Design review of the part built by this model. Coordinates are the model's own, in mm. A direction names the side the tool comes from. Give positions to 0.01 mm unless a question says otherwise; leave off trailing zeros. Loops run counter-clockwise (first coordinate to the right, second up) from the corner with the lowest first, then second, coordinate; pieces in that order, holes last. Notation, with made-up numbers: (44, -17) - (63, -17) arc R24 cw to (63, 4) - close; hole circle Ø6 at (35.25, 85.25). An arc over 180 degrees is marked (long way). Write each question's results on one line, items separated by ' | '.
from build123d import *

# Parameters (mm, degrees)
SKETCH_1_R          = 1.1303
EXTRUDE_1_DEPTH     = 1.588
FILLET_1_R          = 2
FILLET_2_R          = 2
FILLET_3_R          = 2
FILLET_4_R          = 2
SKETCH_2_W          = 12
SKETCH_2_H          = 89.95
EXTRUDE_2_DEPTH     = 1.588
CUT_EXTRUDE_1_DEPTH = 10


with BuildPart() as part:
    # 草图1 → 凸台-拉伸1 (new body)
    with BuildSketch(Plane(origin=(-0.79375, 0, 0), x_dir=(0, -1, 0), z_dir=(-1, 0, 0))):
        with BuildLine():
            Line((38.795, 5), (12.795, 5))
            ThreePointArc((12.795, 5), (11.380786438, 4.414213562), (10.795, 3))
            Line((10.795, 3), (10.795, -13))
            ThreePointArc((10.795, -13), (11.380786438, -14.414213562), (12.795, -15))
            Line((12.795, -15), (47.795, -15))
            Line((47.795, -15), (50.77, -0.039144756))
            Line((50.77, -0.039144756), (55.77, -0.039144756))
            Line((55.77, -0.039144756), (60.77, -0.039144756))
            Line((60.77, -0.039144756), (63.745, -15))
            Line((63.745, -15), (98.745, -15))
            ThreePointArc((98.745, -15), (100.159213562, -14.414213562), (100.745, -13))
            Line((100.745, -13), (100.745, 3))
            ThreePointArc((100.745, 3), (100.159213562, 4.414213562), (98.745, 5))
            Line((98.745, 5), (72.745, 5))
            Line((72.745, 5), (38.795, 5))
        make_face()
        with Locations((18.295, 0)):
            Circle(SKETCH_1_R, mode=Mode.SUBTRACT)
        with Locations((13.295, 0)):
            Circle(SKETCH_1_R, mode=Mode.SUBTRACT)
        with Locations((98.245, 0)):
            Circle(SKETCH_1_R, mode=Mode.SUBTRACT)
        with Locations((93.245, 0)):
            Circle(SKETCH_1_R, mode=Mode.SUBTRACT)
    extrude(amount=-EXTRUDE_1_DEPTH)

    # 圆角1
    fillet_1_edges = [part.edges().sort_by_distance(p)[0] for p in [
        (0.00025, -50.77, -0.039144756),
    ]]
    fillet(fillet_1_edges, radius=FILLET_1_R)

    # 圆角2
    fillet_2_edges = [part.edges().sort_by_distance(p)[0] for p in [
        (0.00025, -47.795, -15),
    ]]
    fillet(fillet_2_edges, radius=FILLET_2_R)

    # 圆角3
    fillet_3_edges = [part.edges().sort_by_distance(p)[0] for p in [
        (0.00025, -60.77, -0.039144756),
    ]]
    fillet(fillet_3_edges, radius=FILLET_3_R)

    # 圆角4
    fillet_4_edges = [part.edges().sort_by_distance(p)[0] for p in [
        (0.00025, -63.745, -15),
    ]]
    fillet(fillet_4_edges, radius=FILLET_4_R)

    # 草图2 → 凸台-拉伸2 (add)
    with BuildSketch(Plane.ZY.offset(0.79375)):
        with Locations((9, -55.77)):
            Rectangle(SKETCH_2_W, SKETCH_2_H)
        Polygon((-25, -10.795), (-25, -45.806477318), (-13.39006724, -48.115138781), (-13, -10.795), align=None)
        Polygon((-13.39006724, -63.424861219), (-25, -65.733522682), (-25, -100.745), (-13, -100.745), align=None)
    extrude(amount=-EXTRUDE_2_DEPTH)

    # 草图5 → 切除-拉伸1 (cut)
    with BuildSketch(Plane(origin=(0.79425, 0, 0), x_dir=(0, 0, -1), z_dir=(1, 0, 0))):
        Polygon((1.649077515, -50.449861219), (25, -45.806477318), (25, -39.241825321), align=None)
        Polygon((25, -72.298174679), (25, -65.733522682), (1.649077515, -61.090138781), align=None)
    extrude(amount=-CUT_EXTRUDE_1_DEPTH, mode=Mode.SUBTRACT)


solid = part.part
(1) Wall thickness on line 1 along Y through (x, z) = (-0.6, -5.5) (3 decimals); line 2 along Y through (x, z) = (0.1, -20) (3 decimals); line 3 along Z through (x, y) = (-0.05, -71): over which ranges is each line inside the solid? List them lowest first. Write a range as from..to.
Answers below:
line 1: -100.745..-62.939, -48.601..-10.795 | line 2: -100.745..-69.898, -41.642..-10.795 | line 3: -22.3..15
(2) Take a section at B-B on z = -13.5. Give the boundary of the cut face in (x, y) (3 decimals).
Answers below:
outline: (-0.794, -100.745) - (0.794, -100.745) - (0.794, -66.778) - (-0.794, -66.778) - close; (-0.794, -44.762) - (0.794, -44.762) - (0.794, -10.795) - (-0.794, -10.795) - close
(3) Tool access review of faces 4 (the flat face through (0.011, -66.616, -13.161)), 5 (the flat face through (0, -86, -25)): name each direction out of +Z, -Z, +X, -X, +Y, -Y from which nothing blocks a thin tool from reaching the whole face with its end or side.
Answers below:
face 4: -Z, +X, -X | face 5: -Z, +X, -X, +Y, -Y
(4) Take a section at A-A on x = 0.2. Give the boundary of the cut face in (y, z) (3 decimals), plus the area to 3 significant figures.
Answers below:
outline: (-100.745, -25) - (-72.298, -25) - (-61.09, -1.649) arc R2 cw to (-59.129, -0.039) - (-52.411, -0.039) arc R2 cw to (-50.45, -1.649) - (-39.242, -25) - (-10.795, -25) - (-10.795, 15) - (-100.745, 15) - close; hole circle Ø2.261 at (-98.245, 0); hole circle Ø2.261 at (-93.245, 0); hole circle Ø2.261 at (-18.295, 0); hole circle Ø2.261 at (-13.295, 0) | area: 3,060 mm2
(5) Draft analysis for pull direction Y (two halves, no side actions). For faces 1 (the cylindrical face through (0.01, -60.38, -0.48)), 2 (the flat face through (0, -10.795, -5)), 3 (the flat face through (0, -56, 15)), state which applies: pulls with the +Y half, pulls with the -Y half, needs draft (parallel to the pull), parting line crosses it, or undercut.
Answers below:
face 1: undercut | face 2: pulls with the +Y half | face 3: needs draft
(6) Insertion check: P1, Ø1.4, axis at y = -93.245, z = 0, coming from the -X side. The pin has a flat end and moves straight along its axis. Give the tip position at first contact, or say it passes through.
Answers below:
P1: through
(7) Take a section at C-C on z = -9. Give the boundary of the cut face in (x, y) (3 decimals).
Answers below:
outline: (-0.794, -100.745) - (0.794, -100.745) - (0.794, -64.618) - (-0.794, -64.618) - close; (-0.794, -46.922) - (0.794, -46.922) - (0.794, -10.795) - (-0.794, -10.795) - close
